Autodesk Inventor part; units mm, degrees
ref_plane "作業平面1" through (0, 1.3, 0) normal (0, 1, 0) x (1, 0, 0)
ref_plane "作業平面2" through (0, -9.9, 0) normal (0, 1, 0) x (1, 0, 0)
ref_plane "作業平面3" through (0, -29.9, 0) normal (0, -1, 0) x (1, 0, 0)
sketch "スケッチ1" plane through (0, 0, 0) normal (0, 1, 0) x (-1, 0, 0)
  circle A0 centre (0, 0) radius 3
  dimension "d0" = 6
extrude "押し出し1" add sketch "スケッチ1" along normal blind 5.2
sketch "スケッチ2" plane through (0, 0, 0) normal (0, -1, 0) x (1, 0, 0)
  circle A0 centre (0, 0) radius 10
  dimension "d3" = 20
extrude "押し出し2" add sketch "スケッチ2" along normal blind 4
sketch "スケッチ3" plane through (0, -4, 0) normal (0, -1, 0) x (1, 0, 0)
  line L0 (0, 0) -> (0, -9.6) construction
  line L1 (10, 10.9) -> (-10, 10.9)
  line L2 (-10, 10.9) -> (-10, -30.1)
  line L3 (-10, -30.1) -> (10, -30.1)
  line L4 (10, -30.1) -> (10, 10.9)
  line L5 (10, 10.9) -> (-10, -30.1) construction
  line L6 (-10, 10.9) -> (10, -30.1) construction
  dimension "d6" = 9.6
  dimension "d7" = 20
  dimension "d8" = 41
extrude "押し出し3" add sketch "スケッチ3" along normal blind 33.8
sketch "スケッチ4" plane through (0, -4, 0) normal (0, 1, 0) x (1, 0, 0)
  circle A0 centre (0, 0) radius 3 construction
  line L0 (0, 0) -> (0, 19.2) construction
  arc A1 (10, 19.2) -> (-10, 19.2) centre (0, 19.2) ccw
  line L1 (-10, 19.2) -> (-10, 0)
  circle A2 centre (0, 0) radius 10 construction
  line L2 (10, 19.2) -> (10, 0)
  line L3 (10, 30.1) -> (10, -10.9)
  arc A3 (10, 0) -> (-10, 0) centre (0, 0) ccw
  dimension "d11" = 19.2
  dimension "d12" = 10
extrude "押し出し4" add sketch "スケッチ4" along normal blind 4
ref_plane "作業平面1" through (0, 1.3, 0) normal (0, 1, 0) x (1, 0, 0)
sketch "スケッチ5" plane through (0, 0, 0) normal (0, 1, 0) x (1, 0, 0)
  circle A0 centre (0, 0) radius 6.25
  dimension "d16" = 12.5
sketch "スケッチ6" plane through (0, 1.3, 0) normal (0, 1, 0) x (1, 0, 0)
  circle A0 centre (0, 0) radius 5.5
  dimension "d17" = 11
loft "ロフト1" add profiles "スケッチ5", "スケッチ6"
ref_plane "作業平面2" through (0, -9.9, 0) normal (0, 1, 0) x (1, 0, 0)
ref_plane "作業平面3" through (0, -29.9, 0) normal (0, -1, 0) x (1, 0, 0)
sketch "スケッチ7" plane through (0, -9.9, 0) normal (0, 1, 0) x (1, 0, 0)
  line L0 (10, -10.9) -> (-10, -10.9)
  line L1 (9, -10.9) -> (-9, -10.9)
  line L2 (-9, -10.9) -> (-9, -18.4)
  line L3 (-9, -18.4) -> (9, -18.4)
  line L4 (9, -18.4) -> (9, -10.9)
  line L5 (10, 30.1) -> (10, -10.9)
  line L6 (9, -15.4) -> (-9, -15.4) construction
  circle A0 centre (5, -15.4) radius 2.35
  circle A1 centre (-5, -15.4) radius 2.35
  point P0 (0, 0)
  dimension "d24" = 18
  dimension "d25" = 7.5
  dimension "d26" = 1
  dimension "d27" = 3
  dimension "d28" = 4.7
  dimension "d29" = 4
  dimension "d30" = 4.7
  dimension "d31" = 4
extrude "押し出し5" add sketch "スケッチ7" along normal blind 2.5
ref_plane "作業平面4" through (10, -4, -9.6) normal (0, 0, -1) x (-1, 0, 0)
mirror "ミラー1" about plane through (10, -4, -9.6) normal (0, 0, -1) of "押し出し5"
sketch "スケッチ8" plane through (0, -29.9, 0) normal (0, -1, 0) x (1, 0, 0)
  line L0 (10, 10.9) -> (-10, 10.9)
  line L1 (9, 10.9) -> (-9, 10.9)
  line L2 (-9, 10.9) -> (-9, 18.4)
  line L3 (-9, 18.4) -> (9, 18.4)
  line L4 (9, 18.4) -> (9, 10.9)
  line L5 (10, -30.1) -> (10, 10.9)
  line L6 (9, 18.4) -> (9, 10.9)
  line L7 (9, 15.4) -> (-9, 15.4) construction
  line L8 (-9, 10.9) -> (-9, 18.4)
  circle A0 centre (5, 15.4) radius 1.6
  circle A1 centre (-5, 15.4) radius 1.6
  point P0 (0, 0)
  dimension "d35" = 18
  dimension "d36" = 7.5
  dimension "d37" = 1
  dimension "d38" = 3
  dimension "d39" = 3.2
  dimension "d40" = 4
  dimension "d41" = 3.2
  dimension "d42" = 4
extrude "押し出し6" add sketch "スケッチ8" along normal blind 2.5
mirror "ミラー2" about plane through (10, -4, -9.6) normal (0, 0, -1) of "押し出し6"
sketch "スケッチ9" plane through (0, -37.8, 0) normal (0, -1, 0) x (1, 0, 0)
  circle A0 centre (0, 0) radius 4
  dimension "d45" = 8
extrude "押し出し7" add sketch "スケッチ9" along normal blind 5.3
sketch "スケッチ10" plane through (0, -37.8, 0) normal (0, -1, 0) x (1, 0, 0)
  circle A0 centre (0, 0) radius 6
  dimension "d48" = 12
extrude "押し出し8" add sketch "スケッチ10" along normal blind 1.3
sketch "スケッチ11" plane through (0, -39.1, 0) normal (0, -1, 0) x (1, 0, 0)
  circle A0 centre (0, 0) radius 5
  dimension "d51" = 10
extrude "押し出し9" add sketch "スケッチ11" along normal blind 0.5
properties part number "krs2350_hv_sa"
Can you work these out from the model? Positions are in its coordinate system, mm. A direction names the side the tool comes from. Give positions to 0.01 mm unless a question says otherwise; leave off trailing zeros. Order: outer loops, then holes, each group sorted by start corner. A loop starts at its lowest first (then second) coordinate and runs counter-clockwise, first axis right, second up. Notation, with made-up numbers: (9, 6.25) - (30, 6.25) arc R25 cw to (30, 22.25) - close; hole circle Ø1 at (-9.5, 85). An arc over 180 degrees is marked (long way). Use a Markdown table: item, result. Add a question column.
Q1. If we section it at C-C on z = 8: Write out the boundary of the cut face in (x, y).
Q2. On a 3-axis mill with a long thin cutter (end or side, diameter ignored), from which of +Z, -Z, +X, -X, +Y, -Y can I reach the whole of each face in a straight line? I mean faces 4 (the flat face through (9, -31, -34)), 5 (the cylindrical face through (-0.2, -2, -29.2)), 6 (the flat face through (-2, -4, 10)). Say none if no direction works.
Q3. If we section it at A-A on z = -34.6: Write out the boundary of the cut face in (x, y).
Q4. If we section it at B-B on y = -31: Write out the boundary of the cut face in (x, z).
Q5. I'm going to push flat-ended pins straight in: pin 1 (1.2 mm diameter, centred on y = -9, z = -33, fed in from +X); pin 2 (5 mm diameter, centred on x = -2.5, y = -15.5, fed in from -Z); pin 3 (3 mm diameter, centred on x = 3, z = -21.5, fed in from +Y). Where does each tip first touch, or does it pass through?
Q6. Please list where these lines run through material, in increasing order: line 1 along Z through (x, y) = (5, -8.05); line 2 along X through (y, z) = (-30, 15.5); line 3 along X through (y, z) = (-9, 15).
Q7. If we section it at D-D on x = -8.25: Write out the boundary of the cut face in (y, z), plus the area to 3 significant figures.
Q8. If we mould it in two halves opening along X, with no side actions, what happens to faces 1 (the cylindrical face through (-0.867, -41.326, 3.905)), 2 (the cylindrical face through (-5.208, -31.132, -36.186)), 3 (the flat face through (-9, -31, -34))? For each: released by +X, released by -X, zero draft, split by the parting line, or undercut.
Answers follow:
| question | item | result |
|---|---|---|
| 1 | outline | (-10, -37.8) - (10, -37.8) - (10, -4) - (6, -4) - (6, 0) - (-6, 0) - (-6, -4) - (-10, -4) - close |
| 2 | face 4 | -Z, +X, +Y, -Y |
| 2 | face 5 | -Z, +Y |
| 2 | face 6 | +Z, +Y |
| 3 | outline | (-9, -32.4) - (-6.6, -32.4) - (-6.6, -29.9) - (-9, -29.9) - close; (-9, -9.9) - (-7.35, -9.9) - (-7.35, -7.4) - (-9, -7.4) - close; (-3.4, -32.4) - (3.4, -32.4) - (3.4, -29.9) - (-3.4, -29.9) - close; (-2.65, -9.9) - (2.65, -9.9) - (2.65, -7.4) - (-2.65, -7.4) - close; (6.6, -32.4) - (9, -32.4) - (9, -29.9) - (6.6, -29.9) - close; (7.35, -9.9) - (9, -9.9) - (9, -7.4) - (7.35, -7.4) - close |
| 4 | outline | (-10, -30.1) - (-9, -30.1) - (-9, -37.6) - (9, -37.6) - (9, -30.1) - (10, -30.1) - (10, 10.9) - (9, 10.9) - (9, 18.4) - (-9, 18.4) - (-9, 10.9) - (-10, 10.9) - close; hole circle Ø3.2 at (-5, -34.6); hole circle Ø3.2 at (-5, 15.4); hole circle Ø3.2 at (5, -34.6); hole circle Ø3.2 at (5, 15.4) |
| 5 | pin 1 | stops at x = 9 |
| 5 | pin 2 | stops at z = -30.1 |
| 5 | pin 3 | stops at y = 0 |
| 6 | line 1 | z = -37.6 to -36.95, -32.25 to 13.05, 17.75 to 18.4 |
| 6 | line 2 | x = -9 to -6.6, -3.4 to 3.4, 6.6 to 9 |
| 6 | line 3 | x = -9 to -7.32, -2.68 to 2.68, 7.32 to 9 |
| 7 | outline | (-37.8, -30.1) - (-32.4, -30.1) - (-32.4, -37.6) - (-29.9, -37.6) - (-29.9, -30.1) - (-9.9, -30.1) - (-9.9, -37.6) - (-7.4, -37.6) - (-7.4, -30.1) - (-4, -30.1) - (-4, -24.85) - (0, -24.85) - (0, 5.65) - (-4, 5.65) - (-4, 10.9) - (-7.4, 10.9) - (-7.4, 18.4) - (-9.9, 18.4) - (-9.9, 10.9) - (-29.9, 10.9) - (-29.9, 18.4) - (-32.4, 18.4) - (-32.4, 10.9) - (-37.8, 10.9) - close |
| 7 | area | 1,580 mm^2 |
| 8 | face 1 | split by the parting line |
| 8 | face 2 | undercut |
| 8 | face 3 | released by -X |
